from build123d import *

# Parameters (mm, degrees)
ESQUISSE1_R        = 12
BOSS_EXTRU_1_DEPTH = 3


with BuildPart() as part:
    # Esquisse1 → Boss.-Extru.1 (new body)
    with BuildSketch(Plane(origin=(0, 0, 0), x_dir=(1, 0, 0), z_dir=(0, 1, 0))):
        Polygon((0, 0), (0, 86.036465453), (9.829824531, 79.153548216), (8.109095222, 76.696092084), (16.300615665, 70.96032772), (18.021344974, 73.417783853), (26.212865417, 67.682019489), (24.492136108, 65.224563357), (32.683656551, 59.488798993), (34.40438586, 61.946255126), (42.595906303, 56.210490762), (40.875176994, 53.75303463), (49.066697437, 48.017270266), (50.787426746, 50.474726399), (58.978947189, 44.738962035), (57.25821788, 42.281505903), (65.449738323, 36.545741539), (67.170467632, 39.003197672), (75.361988075, 33.267433308), (73.641258766, 30.809977175), (81.832779208, 25.074212812), (83.553508517, 27.531668945), (91.74502896, 21.795904581), (90.024299651, 19.338448448), (98.215820094, 13.602684085), (99.936549403, 16.060140218), (108.128069846, 10.324375854), (106.407340537, 7.866919721), (114.59886098, 2.131155358), (116.319590289, 4.588611491), (122.872806643, 0), (122.872806643, -25), (110, -25), (110, -22), (100, -22), (100, -25), (90, -25), (90, -22), (80, -22), (80, -25), (70, -25), (70, -22), (60, -22), (60, -25), (50, -25), (50, -22), (40, -22), (40, -25), (30, -25), (30, -22), (20, -22), (20, -25), (10, -25), (10, -22), (0, -22), align=None)
        with Locations((20, 25.074212812)):
            Circle(ESQUISSE1_R, mode=Mode.SUBTRACT)
    extrude(amount=BOSS_EXTRU_1_DEPTH)


solid = part.part
Here's how the part is built. I have some questions about the finished solid (model axes, mm). A direction names the side the tool comes from. Give positions to 0.01 mm unless a question says otherwise; leave off trailing zeros. Loops run counter-clockwise (first coordinate to the right, second up) from the corner with the lowest first, then second, coordinate; pieces in that order, holes last. Notation, with made-up numbers: (-10.5, 12) -> (9.5, 12) arc R11 ccw to (9.5, 27) -> close; hole circle Ø3 at (57.5, -15.75). An arc over 180 degrees is marked (long way). One line per item, written item: value.
Q1. If I drill on line 1 along X through (y, z) = (1.7, -15); line 2 along X through (y, z) = (1.15, -15.5); line 3 along Z through (x, y) = (57.5, 1.9), over which ranges is the centre line in solid material (lowest first)?
Answers follow:
line 1: 0 to 13.48, 26.52 to 96.22, 99.19 to 101.45
line 2: 0 to 12.77, 27.23 to 95.51, 99.54 to 100.74
line 3: -45.77 to -42.63, -42.11 to 25
Q2. We'd pull the mould along X, two halves only. Please class faces 4 (the face through (65, 1, 22)), 5 (the face through (38.44, 1.48, -59.12)), 6 (the face through (10, 1, 24)): pulls with the +X half, pulls with the -X half, needs draft (parallel to the pull), parting line crosses it, or undercut.
Answers follow:
face 4: undercut
face 5: pulls with the +X half
face 6: pulls with the -X half
Q3. I'm going to push flat-ended pins straight in: pin 1 Ø0.9 at (x, y) = (64, 2) entering from +Z; pin 2 Ø0.9 at (y, z) = (2, 24) entering from -X. Where does each tip first touch, or does it pass through?
Answers follow:
pin 1: z = 22
pin 2: x = 10
Q4. On a 3-axis mill with a long thin cutter (end or side, diameter ignored), from which of +Z, -Z, +X, -X, +Y, -Y can I reach the whole of each face in a straight line? I mean faces 1 (the face through (44.91, 1.48, -50.93)), 2 (the face through (110, 1, 24)), 3 (the face through (5, 1, 22)). Say none if no direction works.
Answers follow:
face 1: +Y, -Y
face 2: +Z, +Y, -Y
face 3: +Z, -X, +Y, -Y
Q5. Suppose I cut it at A-A on z = -69.5. Please give me the cut outline in (x, y), then the cut area to 3 significant figures.
Answers follow:
outline: (0, 0) -> (23.62, 0) -> (23.62, 3) -> (0, 3) -> close
area: 70.8 mm^2
